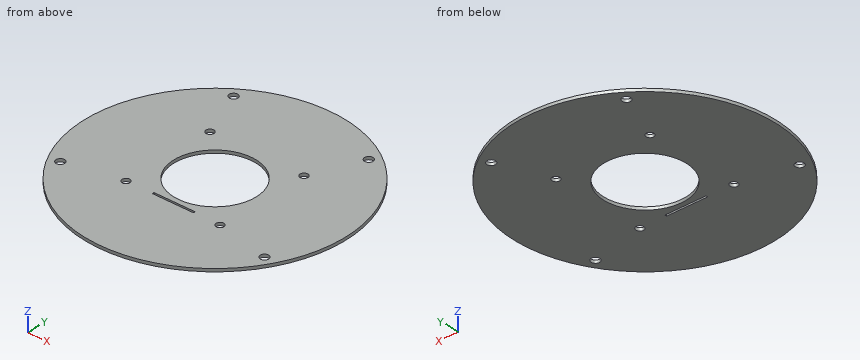
```python
from build123d import *

# Parameters (mm, degrees)
SKETCH3_R              = 53.091965393
SKETCH3_R_2            = 16.75054858
PCB_DEPTH              = 1.2
MAST_REACH             = 77.093
SKETCH5_R              = 1.6
ENCLOSURE_SCREWS_REACH = 77.093
SKETCH6_R              = 1.75
FLEX_CABLE_REACH       = 77.093
SKETCH9_W              = 17
SKETCH9_H              = 0.8


with BuildPart() as part:
    # Sketch3 → PCB (new body)
    with BuildSketch(Plane.XY):
        Circle(SKETCH3_R)
        Circle(SKETCH3_R_2, mode=Mode.SUBTRACT)
    extrude(amount=PCB_DEPTH)

    # Sketch5 → Mast (cut, up to next)
    with BuildSketch(Plane.XY.offset(1.2), mode=Mode.PRIVATE) as mast_sk1:
        with Locations((-19.445436483, -19.445436483)):
            Circle(SKETCH5_R)
    mast_tool1 = extrude(mast_sk1.sketch, amount=-MAST_REACH, mode=Mode.PRIVATE) & part.part
    # Sketch5 → Mast (cut, up to next)
    with BuildSketch(Plane.XY.offset(1.2), mode=Mode.PRIVATE) as mast_sk2:
        with Locations((-19.445436483, 19.445436483)):
            Circle(SKETCH5_R)
    mast_tool2 = extrude(mast_sk2.sketch, amount=-MAST_REACH, mode=Mode.PRIVATE) & part.part
    # Sketch5 → Mast (cut, up to next)
    with BuildSketch(Plane.XY.offset(1.2), mode=Mode.PRIVATE) as mast_sk3:
        with Locations((19.445436483, 19.445436483)):
            Circle(SKETCH5_R)
    mast_tool3 = extrude(mast_sk3.sketch, amount=-MAST_REACH, mode=Mode.PRIVATE) & part.part
    # Sketch5 → Mast (cut, up to next)
    with BuildSketch(Plane.XY.offset(1.2), mode=Mode.PRIVATE) as mast_sk4:
        with Locations((19.445436483, -19.445436483)):
            Circle(SKETCH5_R)
    mast_tool4 = extrude(mast_sk4.sketch, amount=-MAST_REACH, mode=Mode.PRIVATE) & part.part
    add(mast_tool1.solids().sort_by_distance((-19.445436, -19.445436, 1.2))[0], mode=Mode.SUBTRACT)
    add(mast_tool2.solids().sort_by_distance((-19.445436, 19.445436, 1.2))[0], mode=Mode.SUBTRACT)
    add(mast_tool3.solids().sort_by_distance((19.445436, 19.445436, 1.2))[0], mode=Mode.SUBTRACT)
    add(mast_tool4.solids().sort_by_distance((19.445436, -19.445436, 1.2))[0], mode=Mode.SUBTRACT)

    # Sketch6 → Enclosure screws (cut, up to next)
    with BuildSketch(Plane.XY.offset(1.2), mode=Mode.PRIVATE) as enclosure_screws_sk1:
        with Locations((27.960647328, 39.931942749)):
            Circle(SKETCH6_R)
    enclosure_screws_tool1 = extrude(enclosure_screws_sk1.sketch, amount=-ENCLOSURE_SCREWS_REACH, mode=Mode.PRIVATE) & part.part
    # Sketch6 → Enclosure screws (cut, up to next)
    with BuildSketch(Plane.XY.offset(1.2), mode=Mode.PRIVATE) as enclosure_screws_sk2:
        with Locations((42.216920637, -24.373950494)):
            Circle(SKETCH6_R)
    enclosure_screws_tool2 = extrude(enclosure_screws_sk2.sketch, amount=-ENCLOSURE_SCREWS_REACH, mode=Mode.PRIVATE) & part.part
    # Sketch6 → Enclosure screws (cut, up to next)
    with BuildSketch(Plane.XY.offset(1.2), mode=Mode.PRIVATE) as enclosure_screws_sk3:
        with Locations((-42.216920637, -24.373950494)):
            Circle(SKETCH6_R)
    enclosure_screws_tool3 = extrude(enclosure_screws_sk3.sketch, amount=-ENCLOSURE_SCREWS_REACH, mode=Mode.PRIVATE) & part.part
    # Sketch6 → Enclosure screws (cut, up to next)
    with BuildSketch(Plane.XY.offset(1.2), mode=Mode.PRIVATE) as enclosure_screws_sk4:
        with Locations((-27.960647328, 39.931942749)):
            Circle(SKETCH6_R)
    enclosure_screws_tool4 = extrude(enclosure_screws_sk4.sketch, amount=-ENCLOSURE_SCREWS_REACH, mode=Mode.PRIVATE) & part.part
    add(enclosure_screws_tool1.solids().sort_by_distance((27.960647, 39.931943, 1.2))[0], mode=Mode.SUBTRACT)
    add(enclosure_screws_tool2.solids().sort_by_distance((42.216921, -24.37395, 1.2))[0], mode=Mode.SUBTRACT)
    add(enclosure_screws_tool3.solids().sort_by_distance((-42.216921, -24.37395, 1.2))[0], mode=Mode.SUBTRACT)
    add(enclosure_screws_tool4.solids().sort_by_distance((-27.960647, 39.931943, 1.2))[0], mode=Mode.SUBTRACT)

    # Sketch9 → Flex cable (cut, up to next)
    with BuildSketch(Plane.XY, mode=Mode.PRIVATE) as flex_cable_sk1:
        with Locations((0, -19.15054858)):
            Rectangle(SKETCH9_W, SKETCH9_H)
    flex_cable_tool1 = extrude(flex_cable_sk1.sketch, amount=FLEX_CABLE_REACH, mode=Mode.PRIVATE) & part.part
    add(flex_cable_tool1.solids().sort_by_distance((0, -19.150549, 0))[0], mode=Mode.SUBTRACT)


solid = part.part
```
The listing builds one solid part. Answer for the finished solid, in the listing's coordinates (mm). Give positions to 0.01 mm unless a question says otherwise; leave off trailing zeros. Loops run counter-clockwise (first coordinate to the right, second up) from the corner with the lowest first, then second, coordinate; pieces in that order, holes last. Notation, with made-up numbers: (24, -32.5) - (71, -32.5) arc R31 ccw to (71, -6.5) - close; hole circle Ø9 at (-31, 58). An arc over 180 degrees is marked (long way). Return JSON: item names as keys, results as strings. Group by question number.
1. Find section A-A (x = 0). Write down the section's boundary in (y, z), then the cut area to 3 significant figures.
2. Find section C-C (z = 0.85). State how many separate pieces and enclosed holes the cut face has, then the cut area to 3 significant figures.
3. Given pin 1 Ø3 at (x, y) = (-27.96, 39.93) entering from +Z; pin 2 Ø0.6 at (y, z) = (-19, 1) entering from -X, each flat-ended and moving along its own axis, determine where each tip first touches the part or whether it passes through.
4. Straight lines are drawn through the part: line 1 (Y direction, x = 0, z = 0.95); line 2 (X direction, y = 20, z = 0.55); line 3 (X direction, y = -0.5, z = 0.25). For each, find the intervals that lie inside material, in ascending order. Write a range as [from, to].
5. Find section D-D (x = -31). Write down the section's boundary in (y, z).
6. Find section B-B (y = 3). Write down the section's boundary in (x, z).
Verdict:
{
 "1": {"outline": "(-53.09, 0) - (-19.55, 0) - (-19.55, 1.2) - (-53.09, 1.2) - close; (-18.75, 0) - (-16.75, 0) - (-16.75, 1.2) - (-18.75, 1.2) - close; (16.75, 0) - (53.09, 0) - (53.09, 1.2) - (16.75, 1.2) - close", "area": "86.3 mm^2"},
 "2": {"separate pieces": "1", "enclosed holes": "10", "area": "7,890 mm^2"},
 "3": {"pin 1": "passes through", "pin 2": "stops at x = -49.69"},
 "4": {"line 1": "y = [-53.09, -19.55], [-18.75, -16.75], [16.75, 53.09]", "line 2": "x = [-49.18, -20.95], [-17.94, 17.94], [20.95, 49.18]", "line 3": "x = [-53.09, -16.74], [16.74, 53.09]"},
 "5": {"outline": "(-43.1, 0) - (43.1, 0) - (43.1, 1.2) - (-43.1, 1.2) - close"},
 "6": {"outline": "(-53.01, 0) - (-16.48, 0) - (-16.48, 1.2) - (-53.01, 1.2) - close; (16.48, 0) - (53.01, 0) - (53.01, 1.2) - (16.48, 1.2) - close"}
}
